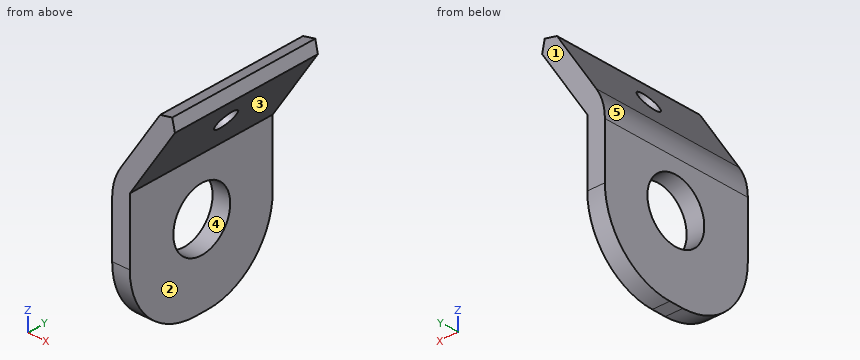
from build123d import *

# Parameters (mm, degrees)
F1_DEPTH    = 44
F2_R        = 15
F3_T1_DEPTH = 69.7168298797
F4_R        = 20
F5_R        = 8.75
F6_DEPTH    = 25
F7_R        = 3.25
F8_DEPTH    = 25


# Not quite as in the source:
# - a fillet or chamfer that OpenCascade refuses, or shapes differently, is made with other operations: its cross-section is extruded or revolved along the edge and cut away or added


with BuildPart() as f1:
    # F0 (on Front) → F1 (new body)
    with BuildSketch(Plane.XZ):
        Polygon((29.4669866014, 53.6632488984), (13.1538538262, 28.4862415493), (13.1538538262, -11.5137584507), (18.1538538262, -11.5137584507), (18.1538538262, 27.0079869683), (33.6631544929, 50.9443934359), align=None)
    extrude(amount=F1_DEPTH)

    # F2
    f2_edges = [f1.edges().sort_by_distance(p)[0] for p in [
        (13.153854, -22, 28.486242),
    ]]
    fillet(f2_edges, radius=F2_R)

    # F3: chamfer of 5 on 2 edges, made by hand

    # F3_s2 → F3_t1 (cut)
    with BuildSketch(Plane.XZ.offset(-12.8584149398)):
        Polygon((26.7481311389, 49.4670810069), (33.6631544929, 50.9443934359), (29.4669866014, 53.6632488984), align=None)
        Polygon((29.4669866014, 53.6632488984), (30.9442990304, 46.7482255444), (33.6631544929, 50.9443934359), align=None)
    extrude(amount=F3_T1_DEPTH, mode=Mode.SUBTRACT)

    # F4
    f4_edges = [f1.edges().sort_by_distance(p)[0] for p in [
        (15.653854, -44, -11.513758),
        (15.653854, 0, -11.513758),
    ]]
    fillet(f4_edges, radius=F4_R)

    # F5 (on face) → F6 (cut)
    with BuildSketch(Plane.YZ.offset(18.1538538262)):
        with Locations((-21.8509025872, 11.1763291061)):
            Circle(F5_R)
    extrude(amount=-F6_DEPTH, mode=Mode.SUBTRACT)

    # F7 (on face) → F8 (cut)
    with BuildSketch(Plane(origin=(0.4608744572, 0, -0.2986179457), x_dir=(0, 1, 0), z_dir=(0.8392335783, 0, -0.5437710925))):
        with Locations((-22.313432768, 45.9909811616)):
            Circle(F7_R)
    extrude(amount=-F8_DEPTH, mode=Mode.SUBTRACT)


solid = f1.part
Can you work these out from the model? Positions are in its coordinate system, mm. Face numbers are marked on the shaded views. A direction names the side the tool comes from. Give positions to 0.01 mm unless a question says otherwise; leave off trailing zeros. Order: outer loops, then holes, each group sorted by start corner. A loop starts at its lowest first (then second) coordinate and runs counter-clockwise, first axis right, second up. Notation, with made-up numbers: M 61.5,-3 L 89.5,-3 A23 cw 89.5,25 Z; hole C -24,6.25 d1. An arc over 180 degrees is marked long. One line per item, written item: value.
Item 1: For the marked faces 1 and 2, which set-ups out of +Z, -Z, +X, -X, +Y, -Y let a thin tool reach every point of the face, with its end or its side?
Verdict:
face 1: +Z, -Z, +X, -X, +Y
face 2: -Z, +X, +Y, -Y
Item 2: If we section it at C-C on x = 17.5: Write out the boundary of the cut face in (y, z).
Verdict:
outline: M -44,8.49 A20 ccw -24,-11.51 L -20,-11.51 A20 ccw 0,8.49 L 0,35.19 L -44,35.19 Z; hole C -21.85,11.18 d17.5
Item 3: For pin 1 (23 mm diameter, centred on y = -21.85, z = 11.18, fed in from -X); pin 2 (11.5 mm diameter, centred on y = -28.5, z = 5, fed in from +X); pin 3 (6 mm diameter, centred on y = -17.5, z = 14.5, fed in from +X); pin 4 (8 mm diameter, centred on x = 20, y = -28, fed in from +Z), each with a flat end and sliding along its axis, tell me the tip position at first contact or that it passes through.
Verdict:
pin 1: x = 13.15
pin 2: x = 18.15
pin 3: through
pin 4: z = 45.23
Item 4: If we section it at B-B on z = 17: Write out the boundary of the cut face in (x, y), and give its area (3 significant figures).
Verdict:
outline: M 13.15,-44 L 18.15,-44 L 18.15,-28.38 L 13.15,-28.38 Z; M 13.15,-15.32 L 18.15,-15.32 L 18.15,0 L 13.15,0 Z
area: 155 mm2
Item 5: Please list where these lines run through material, in increasing order: line 1 (X direction, y = -10.5, z = 0); line 2 (Z direction, x = 30, y = -39); line 3 (Z direction, x = 26.5, y = -36).
Verdict:
line 1: 13.15 to 18.15
line 2: 45.29 to 50.16
line 3: 39.89 to 49.08
Item 6: If we mould it in two halves opening along Z, with no side actions, what happens to the marked faces 3, 4 and 5? For each: pulls with the +Z half, pulls with the -Z half, needs draft (parallel to the pull), parting line crosses it, or undercut.
Verdict:
face 3: pulls with the -Z half
face 4: undercut
face 5: pulls with the +Z half
Item 7: If we section it at A-A on y = -21.5: Write out the boundary of the cut face in (x, z).
Verdict:
outline: M 13.15,-11.51 L 18.15,-11.51 L 18.15,2.43 L 13.15,2.43 Z; M 13.15,19.92 L 18.15,19.92 L 18.15,27.01 L 23.76,35.66 L 19.56,38.38 L 15.57,32.21 A15 ccw 13.15,24.05 Z; M 22.98,43.66 L 27.18,40.94 L 30.94,46.75 L 30.21,50.21 L 26.75,49.47 Z
Item 8: If we section it at D-D on y = -7: Write out the boundary of the cut face in (x, z).
Verdict:
outline: M 13.15,-6.71 L 18.15,-6.71 L 18.15,27.01 L 30.94,46.75 L 30.21,50.21 L 26.75,49.47 L 15.57,32.21 A15 ccw 13.15,24.05 Z
